Model file for the job. Use its own axes, mm. Face numbers are marked on the shaded views. A direction names the side the tool comes from. Coordinates: 2 decimals unless noted, no trailing zeros. Order: outer loops, then holes, each group sorted by start corner. A loop starts at its lowest first (then second) coordinate and runs counter-clockwise, first axis right, second up. Notation, with made-up numbers: M -8,3 L 43,3 A21 cw 43,28 Z; hole C 83,46 d11. An arc over 180 degrees is marked long. Return JSON: item names as keys, results as strings.
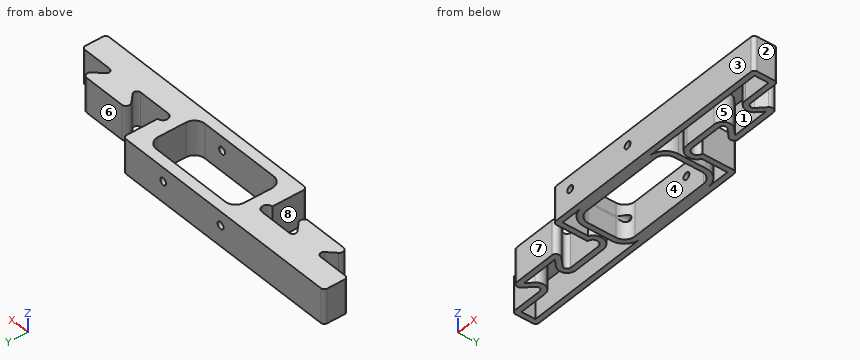
```python
from build123d import *

# Parameters (mm, degrees)
ABS_ZWING_MIRRORED_START      = -10
ABS_ZWING_MIRRORED_DEPTH      = 10
ABS_ZWING_MIRRORED_START_2    = -1.5
ABS_ZWING_MIRRORED_2_DEPTH    = 1.5
SKETCH1_W                     = 30
SKETCH1_H                     = 14
CUT_EXTRUDE1_DEPTH            = 10
FILLET1_R                     = 3
BOSS_EXTRUDE2_DEPTH           = 8.5
CUT_EXTRUDE2_DEPTH            = 10
TAP_DRILL_FOR_M2_5_TAP1_D     = 2.05
TAP_DRILL_FOR_M2_5_TAP1_DEPTH = 30.5


# Read off the part's stored shape, not the designer's step: abs_zwing_Mirrored
with BuildPart() as part:
    # abs_zwing_Mirrored outline → abs_zwing_Mirrored (new body)
    with BuildSketch(Plane.XY.offset(ABS_ZWING_MIRRORED_START)):
        with BuildLine():
            ThreePointArc((-23.5, 2.5), (-22, 1), (-23.5, -0.5))
            Line((-23.5, -0.5), (-23.5, -9.5))
            ThreePointArc((-23.5, -9.5), (-23.207106781, -10.207106781), (-22.5, -10.5))
            Line((-22.5, -10.5), (45.5, -10.5))
            ThreePointArc((45.5, -10.5), (46.207106781, -10.207106781), (46.5, -9.5))
            Line((46.5, -9.5), (46.5, -4.5))
            ThreePointArc((46.5, -4.5), (46.207106781, -3.792893219), (45.5, -3.5))
            Line((45.5, -3.5), (36.914213562, -3.5))
            ThreePointArc((36.914213562, -3.5), (35.99033403, -2.882683432), (36.207106781, -1.792893219))
            Line((36.207106781, -1.792893219), (38.792893219, 0.792893219))
            ThreePointArc((38.792893219, 0.792893219), (39.00966597, 1.882683432), (38.085786438, 2.5))
            Line((38.085786438, 2.5), (24.914213562, 2.5))
            ThreePointArc((24.914213562, 2.5), (23.99033403, 1.882683432), (24.207106781, 0.792893219))
            Line((24.207106781, 0.792893219), (26.792893219, -1.792893219))
            ThreePointArc((26.792893219, -1.792893219), (27.00966597, -2.882683432), (26.085786438, -3.5))
            Line((26.085786438, -3.5), (16.5, -3.5))
            ThreePointArc((16.5, -3.5), (15, -2), (16.5, -0.5))
            Line((16.5, -0.5), (16.5, 8.5))
            ThreePointArc((16.5, 8.5), (16.207106781, 9.207106781), (15.5, 9.5))
            Line((15.5, 9.5), (-52.5, 9.5))
            ThreePointArc((-52.5, 9.5), (-53.207106781, 9.207106781), (-53.5, 8.5))
            Line((-53.5, 8.5), (-53.5, 3.5))
            ThreePointArc((-53.5, 3.5), (-53.207106781, 2.792893219), (-52.5, 2.5))
            Line((-52.5, 2.5), (-43.914213562, 2.5))
            ThreePointArc((-43.914213562, 2.5), (-42.99033403, 1.882683432), (-43.207106781, 0.792893219))
            Line((-43.207106781, 0.792893219), (-45.792893219, -1.792893219))
            ThreePointArc((-45.792893219, -1.792893219), (-46.00966597, -2.882683432), (-45.085786438, -3.5))
            Line((-45.085786438, -3.5), (-31.914213562, -3.5))
            ThreePointArc((-31.914213562, -3.5), (-30.99033403, -2.882683432), (-31.207106781, -1.792893219))
            Line((-31.207106781, -1.792893219), (-33.792893219, 0.792893219))
            ThreePointArc((-33.792893219, 0.792893219), (-34.00966597, 1.882683432), (-33.085786438, 2.5))
            Line((-33.085786438, 2.5), (-23.5, 2.5))
        make_face()
        with BuildLine():
            ThreePointArc((-22, -1.598076211), (-20.602222521, 1.776457136), (-23.5, 4))
            Line((-23.5, 4), (-33.085786438, 4))
            ThreePointArc((-33.085786438, 4), (-35.395485269, 2.456708581), (-34.853553391, -0.267766953))
            Line((-34.853553391, -0.267766953), (-33.121320344, -2))
            Line((-33.121320344, -2), (-43.878679656, -2))
            Line((-43.878679656, -2), (-42.146446609, -0.267766953))
            ThreePointArc((-42.146446609, -0.267766953), (-41.604514731, 2.456708581), (-43.914213562, 4))
            Line((-43.914213562, 4), (-52, 4))
            Line((-52, 4), (-52, 8))
            Line((-52, 8), (15, 8))
            Line((15, 8), (15, 0.598076211))
            ThreePointArc((15, 0.598076211), (13.602222521, -2.776457136), (16.5, -5))
            Line((16.5, -5), (26.085786438, -5))
            ThreePointArc((26.085786438, -5), (28.395485269, -3.456708581), (27.853553391, -0.732233047))
            Line((27.853553391, -0.732233047), (26.121320344, 1))
            Line((26.121320344, 1), (36.878679656, 1))
            Line((36.878679656, 1), (35.146446609, -0.732233047))
            ThreePointArc((35.146446609, -0.732233047), (34.604514731, -3.456708581), (36.914213562, -5))
            Line((36.914213562, -5), (45, -5))
            Line((45, -5), (45, -9))
            Line((45, -9), (-22, -9))
            Line((-22, -9), (-22, -1.598076211))
        make_face(mode=Mode.SUBTRACT)
    extrude(amount=ABS_ZWING_MIRRORED_DEPTH)

    # abs_zwing_Mirrored 2 outline → abs_zwing_Mirrored 2 (add)
    with BuildSketch(Plane.XY.offset(ABS_ZWING_MIRRORED_START_2)):
        with BuildLine():
            Line((-33.085786438, 4), (-23.5, 4))
            ThreePointArc((-23.5, 4), (-20.602222521, 1.776457136), (-22, -1.598076211))
            Line((-22, -1.598076211), (-22, -9))
            Line((-22, -9), (45, -9))
            Line((45, -9), (45, -5))
            Line((45, -5), (36.914213562, -5))
            ThreePointArc((36.914213562, -5), (34.604514731, -3.456708581), (35.146446609, -0.732233047))
            Line((35.146446609, -0.732233047), (36.878679656, 1))
            Line((36.878679656, 1), (26.121320344, 1))
            Line((26.121320344, 1), (27.853553391, -0.732233047))
            ThreePointArc((27.853553391, -0.732233047), (28.395485269, -3.456708581), (26.085786438, -5))
            Line((26.085786438, -5), (16.5, -5))
            ThreePointArc((16.5, -5), (13.602222521, -2.776457136), (15, 0.598076211))
            Line((15, 0.598076211), (15, 8))
            Line((15, 8), (-52, 8))
            Line((-52, 8), (-52, 4))
            Line((-52, 4), (-43.914213562, 4))
            ThreePointArc((-43.914213562, 4), (-41.604514731, 2.456708581), (-42.146446609, -0.267766953))
            Line((-42.146446609, -0.267766953), (-43.878679656, -2))
            Line((-43.878679656, -2), (-33.121320344, -2))
            Line((-33.121320344, -2), (-34.853553391, -0.267766953))
            ThreePointArc((-34.853553391, -0.267766953), (-35.395485269, 2.456708581), (-33.085786438, 4))
        make_face()
    extrude(amount=ABS_ZWING_MIRRORED_2_DEPTH)

    # Sketch1 → Cut-Extrude1 (cut)
    with BuildSketch(Plane(origin=(0, 0, -1.5), x_dir=(-1, 0, 0), z_dir=(0, 0, -1))):
        with Locations((3.5, -0.5)):
            Rectangle(SKETCH1_W, SKETCH1_H)
    extrude(amount=-CUT_EXTRUDE1_DEPTH, mode=Mode.SUBTRACT)

    # Fillet1
    fillet1_edges = [part.edges().sort_by_distance(p)[0] for p in [
        (11.5, -7.5, -0.75),
        (11.5, 6.5, -0.75),
        (-18.5, 6.5, -0.75),
        (-18.5, -7.5, -0.75),
    ]]
    fillet(fillet1_edges, radius=FILLET1_R)

    # Sketch4 → Boss-Extrude2 (add)
    with BuildSketch(Plane(origin=(0, 0, -1.5), x_dir=(-1, 0, 0), z_dir=(0, 0, -1))):
        with BuildLine():
            Line((-13, 3.5), (-13, -4.5))
            ThreePointArc((-13, -4.5), (-11.681980515, -7.681980515), (-8.5, -9))
            Line((-8.5, -9), (15.5, -9))
            ThreePointArc((15.5, -9), (18.681980515, -7.681980515), (20, -4.5))
            Line((20, -4.5), (20, 3.5))
            ThreePointArc((20, 3.5), (18.681980515, 6.681980515), (15.5, 8))
            Line((15.5, 8), (-8.5, 8))
            ThreePointArc((-8.5, 8), (-11.681980515, 6.681980515), (-13, 3.5))
        make_face()
        with BuildLine():
            Line((-11.5, 3.5), (-11.5, -4.5))
            ThreePointArc((-11.5, -4.5), (-10.621320344, -6.621320344), (-8.5, -7.5))
            Line((-8.5, -7.5), (15.5, -7.5))
            ThreePointArc((15.5, -7.5), (17.621320344, -6.621320344), (18.5, -4.5))
            Line((18.5, -4.5), (18.5, 3.5))
            ThreePointArc((18.5, 3.5), (17.621320344, 5.621320344), (15.5, 6.5))
            Line((15.5, 6.5), (-8.5, 6.5))
            ThreePointArc((-8.5, 6.5), (-10.621320344, 5.621320344), (-11.5, 3.5))
        make_face(mode=Mode.SUBTRACT)
    extrude(amount=BOSS_EXTRUDE2_DEPTH)

    # Sketch8 → Cut-Extrude2 (cut)
    with BuildSketch(Plane(origin=(0, 0, -10), x_dir=(-1, 0, 0), z_dir=(0, 0, -1))):
        with BuildLine():
            Line((-38.451471863, 0.451471863), (-40.5, 2.5))
            Line((-40.5, 2.5), (-37.602943725, 2.5))
            ThreePointArc((-37.602943725, 2.5), (-38.711599164, 1.759220119), (-38.451471863, 0.451471863))
        make_face()
        with BuildLine():
            Line((-25.397056275, 2.5), (-22.5, 2.5))
            Line((-22.5, 2.5), (-24.548528137, 0.451471863))
            ThreePointArc((-24.548528137, 0.451471863), (-24.288400836, 1.759220119), (-25.397056275, 2.5))
        make_face()
        with BuildLine():
            Line((33, 0), (31.548528137, -1.451471863))
            ThreePointArc((31.548528137, -1.451471863), (31.288400836, -2.759220119), (32.397056275, -3.5))
            Line((32.397056275, -3.5), (44.602943725, -3.5))
            ThreePointArc((44.602943725, -3.5), (45.711599164, -2.759220119), (45.451471863, -1.451471863))
            Line((45.451471863, -1.451471863), (44.329289322, -0.329289322))
            Line((44.329289322, -0.329289322), (49.897345602, -0.329289322))
            Line((49.897345602, -0.329289322), (49.897345602, -5.77544861))
            Line((49.897345602, -5.77544861), (28.682020132, -5.77544861))
            Line((28.682020132, -5.77544861), (28.682020132, 0))
            Line((28.682020132, 0), (33, 0))
        make_face()
    extrude(amount=-CUT_EXTRUDE2_DEPTH, mode=Mode.SUBTRACT)

    # Tap Drill for M2.5 Tap1
    with Locations(Plane.XZ.offset(10.5)):
        with Locations((-17.5, -4), (2.5, -4)):
            Hole(TAP_DRILL_FOR_M2_5_TAP1_D / 2, depth=TAP_DRILL_FOR_M2_5_TAP1_DEPTH)


solid = part.part
```
Item 1: Saw through at C-C (z = -6). Count the separate pieces of the cut face and the enclosed holes in it, and give its area (3 significant figures).
Check result:
{"separate pieces": "1", "enclosed holes": "3", "area": "538 mm2"}
Item 2: Wall check: line 1 (Y direction, x = -44, z = -1.75); line 2 (Y direction, x = -13.5, z = -2); line 3 (Z direction, x = -17.5, y = -9.25) (3 decimals). Give the ranges that are in metal, low to high.
Check result:
{"line 1": "y = -3.5 to 0, 2.5 to 4, 8 to 9.5", "line 2": "y = -10.5 to -7.5, 6.5 to 9.5", "line 3": "z = -10 to -5.025, -2.975 to 0"}
Item 3: Drop flat-ended pins along their axis: pin 1 Ø1.6 at (x, z) = (2.5, -4) entering from -Y; pin 2 Ø4 at (y, z) = (1, -2) entering from +X; pin 3 Ø2.5 at (y, z) = (-1.5, -5) entering from -X; pin 4 Ø2 at (y, z) = (-6.5, -5.5) entering from -X. Give the stop position or say it passes through.
Check result:
{"pin 1": "passes through", "pin 2": "stops at x = 38.8", "pin 3": "stops at x = -45.8", "pin 4": "stops at x = -23.5"}
Item 4: 3-axis set-ups, long thin cutter, end or side, ignore diameter. For the marked faces 4, 5, 6, 7 and 8: which of +Z, -Z, +X, -X, +Y, -Y reach the whole face in a straight line?
Check result:
{"face 4": "+Z, -Z", "face 5": "-Z", "face 6": "+Z, -Z, +X, +Y", "face 7": "+Z, -Z, -X, -Y", "face 8": "+Z, -Z, -Y"}
Item 5: Pull direction Y, two halves, no side cores. Call the marked faces 1, 2 and 3: +Y half, -Y half, draft (parallel to the pull), parting line (faces both ways), or undercut.
Check result:
{"face 1": "undercut", "face 2": "draft", "face 3": "-Y half"}
Item 6: Saw through at A-A (x = 2.5). Write the cut outline in (y, z) (3 decimals).
Check result:
{"outline": "M -10.5,-10 L -7.5,-10 L -7.5,-5.025 L -10.5,-5.025 Z; M -10.5,-2.975 L -7.5,-2.975 L -7.5,0 L -10.5,0 Z; M 6.5,-10 L 9.5,-10 L 9.5,-5.025 L 6.5,-5.025 Z; M 6.5,-2.975 L 9.5,-2.975 L 9.5,0 L 6.5,0 Z"}
Item 7: Saw through at D-D (x = -39.5). Write the cut outline in (y, z), and give its area (3 significant figures).
Check result:
{"outline": "M -3.5,-10 L -2,-10 L -2,-1.5 L 8,-1.5 L 8,-10 L 9.5,-10 L 9.5,0 L -3.5,0 Z", "area": "45.0 mm2"}
Item 8: Saw through at B-B (x = -26). Write the cut outline in (y, z).
Check result:
{"outline": "M 2.5,-10 L 4,-10 L 4,-1.5 L 8,-1.5 L 8,-10 L 9.5,-10 L 9.5,0 L 2.5,0 Z"}
